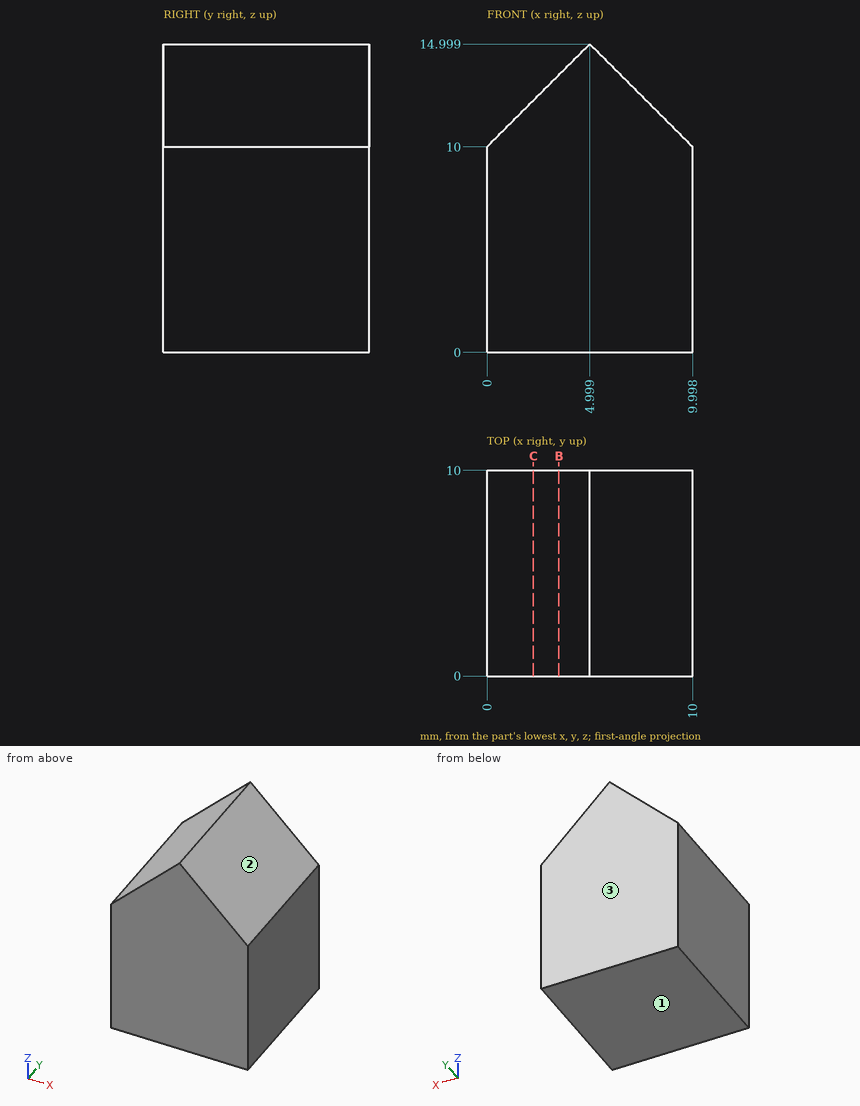
Part print with two shaded views. Sizes in mm from the minimum x, y, z corner. Round coordinates to 2 decimals unless told otherwise and drop trailing zeros. Order: outer loops, then holes, each group sorted by start corner. A loop starts at its lowest first (then second) coordinate and runs counter-clockwise, first axis right, second up.
(1) Pull direction Z, two halves, no side cores. Call the marked faces 1, 2 and 3: released by +Z, released by -Z, zero draft, split by the parting line, or undercut.
(2) Drill centre lines: line 1 (Z direction, x = 1.25, y = 5); line 2 (X direction, y = 2, z = 11.75); line 3 (Z direction, x = 9.5, y = 4.25). Where is each one in solid material? Low to high.
(3) Band-saw the part on C-C (x = 2.25). List the corners of the cut face in (y, z), then the cut area to 4 significant figures.
(4) Pin check, flat tips, straight feed: pin 1 (3 mm diameter, centred on y = 6.5, z = 12.5, fed in from -X); pin 2 (1.5 mm diameter, centred on y = 4.5, z = 13.5, fed in from +X). Stop position of each tip, or through.
(5) Band-saw the part on B-B (x = 3.5). List the corners of the cut face in (y, z), then the cut area to 3 significant figures.
Verdict:
1. face 1: released by -Z
1. face 2: released by +Z
1. face 3: zero draft
2. line 1: z = 0 to 11.25
2. line 2: x = 1.75 to 8.25
2. line 3: z = 0 to 10.5
3. outline: (0, 0) - (10, 0) - (10, 12.25) - (0, 12.25) - close
3. area: 122.5 mm2
4. pin 1: stops at x = 1
4. pin 2: stops at x = 7.25
5. outline: (0, 0) - (10, 0) - (10, 13.5) - (0, 13.5) - close
5. area: 135 mm2
